Source: CAD feature listing. Evaluate the final solid. Frame: model axes, mm. Face numbers are marked on the shaded views. A direction names the side the tool comes from. Coordinates: 2 decimals unless noted, no trailing zeros. Write each loop counter-clockwise with the first axis right and the second up, starting at its lowest first coordinate (ties: lowest second). Pieces come first, ordered by that corner, then holes. Notation, with made-up numbers: (49.25, 35.25) - (95.25, 35.25) arc R18 cw to (95.25, 58.25) - close; hole circle Ø1 at (25.5, 40.25). An arc over 180 degrees is marked (long way). One line per item, written item: value.
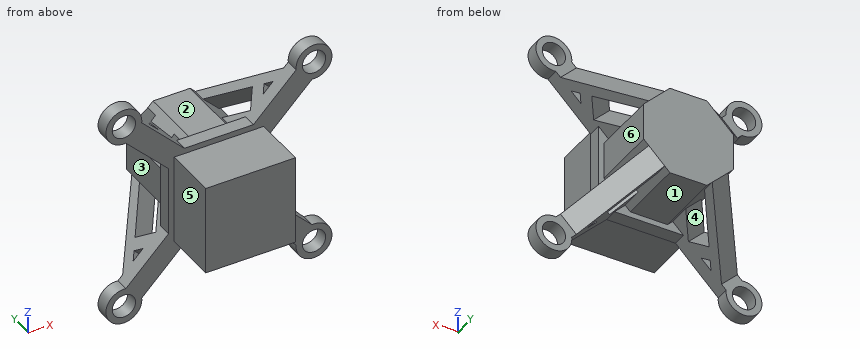
from build123d import *

# Parameters (mm, degrees)
SKETCH1_W               = 20
SKETCH1_H               = 20
BOSS_EXTRUDE1_DEPTH     = 12
BOSS_EXTRUDE2_DEPTH     = 3
BOSS_EXTRUDE3_DEPTH     = 15
BOSS_EXTRUDE4_DEPTH     = 15
BODY_MOVE_COPY1_ANGLE   = 45
CUT_EXTRUDE2_DEPTH      = 15
CUT_EXTRUDE2_DEPTH_BACK = 15
CUT_EXTRUDE3_DEPTH      = 15
CUT_EXTRUDE3_DEPTH_BACK = 15
CUT_EXTRUDE4_DEPTH      = 15
CUT_EXTRUDE4_DEPTH_BACK = 15
CUT_EXTRUDE5_DEPTH      = 15
CUT_EXTRUDE5_DEPTH_BACK = 15
SKETCH10_R              = 2.6
CUT_EXTRUDE6_DEPTH      = 25
BODY_MOVE_COPY2_ANGLE   = 45


with BuildPart() as part:
    # Sketch1 → Boss-Extrude1 (new body)
    with BuildSketch(Plane(origin=(0, 0, 0), x_dir=(1, 0, 0), z_dir=(0, 1, 0))):
        Rectangle(SKETCH1_W, SKETCH1_H)
    extrude(amount=-BOSS_EXTRUDE1_DEPTH)

    # Sketch2 → Boss-Extrude2 (add)
    with BuildSketch(Plane(origin=(0, 0, 0), x_dir=(1, 0, 0), z_dir=(0, 1, 0))):
        with BuildLine():
            Line((7.714466094, -11.25), (17.237496266, -20.773030172))
            ThreePointArc((17.237496266, -20.773030172), (24.04163056, -24.04163056), (20.773030172, -17.237496266))
            Line((20.773030172, -17.237496266), (11.25, -7.714466094))
            Line((11.25, -7.714466094), (11.25, 7.714466094))
            Line((11.25, 7.714466094), (20.773030172, 17.237496266))
            ThreePointArc((20.773030172, 17.237496266), (24.04163056, 24.04163056), (17.237496266, 20.773030172))
            Line((17.237496266, 20.773030172), (7.714466094, 11.25))
            Line((7.714466094, 11.25), (-7.714466094, 11.25))
            Line((-7.714466094, 11.25), (-17.237496266, 20.773030172))
            ThreePointArc((-17.237496266, 20.773030172), (-24.04163056, 24.04163056), (-20.773030172, 17.237496266))
            Line((-20.773030172, 17.237496266), (-11.25, 7.714466094))
            Line((-11.25, 7.714466094), (-11.25, -7.714466094))
            Line((-11.25, -7.714466094), (-20.773030172, -17.237496266))
            ThreePointArc((-20.773030172, -17.237496266), (-24.04163056, -24.04163056), (-17.237496266, -20.773030172))
            Line((-17.237496266, -20.773030172), (-7.714466094, -11.25))
            Line((-7.714466094, -11.25), (7.714466094, -11.25))
        make_face()
    extrude(amount=BOSS_EXTRUDE2_DEPTH)

    # Sketch3 → Boss-Extrude3 (add)
    with BuildSketch(Plane(origin=(0, 3, 0), x_dir=(1, 0, 0), z_dir=(0, 1, 0))):
        Polygon((10, 4.142135624), (4.142135624, 10), (-4.142135624, 10), (-10, 4.142135624), (-10, -4.142135624), (-4.142135624, -10), (4.142135624, -10), (10, -4.142135624), align=None)
    extrude(amount=BOSS_EXTRUDE3_DEPTH)

    # Sketch4 → Boss-Extrude4 (add)
    with BuildSketch(Plane(origin=(0, 3, 0), x_dir=(1, 0, 0), z_dir=(0, 1, 0))):
        Polygon((-11.25, -7.714466094), (-19.735281374, -16.199747468), (-16.199747468, -19.735281374), (-7.714466094, -11.25), (-5.303300859, -8.838834765), (-8.838834765, -5.303300859), align=None)
        Polygon((-7.714466094, 11.25), (-16.199747468, 19.735281374), (-19.735281374, 16.199747468), (-11.25, 7.714466094), (-8.838834765, 5.303300859), (-5.303300859, 8.838834765), align=None)
        Polygon((11.25, 7.714466094), (19.735281374, 16.199747468), (16.199747468, 19.735281374), (7.714466094, 11.25), (5.303300859, 8.838834765), (8.838834765, 5.303300859), align=None)
        Polygon((7.714466094, -11.25), (16.199747468, -19.735281374), (19.735281374, -16.199747468), (11.25, -7.714466094), (8.838834765, -5.303300859), (5.303300859, -8.838834765), align=None)
    extrude(amount=BOSS_EXTRUDE4_DEPTH)


with BuildPart() as part_1:
    # Body-Move/Copy1: moved
    add(part.part.rotate(Axis((0, 0, 0), (0, 1, 0)), BODY_MOVE_COPY1_ANGLE))

    # Sketch5 → Cut-Extrude2 (cut, two sides: drawn at the far end of the back side and taken through both)
    with BuildSketch(Plane.XY.offset(-CUT_EXTRUDE2_DEPTH_BACK)):
        Polygon((-25.409902577, 18), (-10, 18), (-25.409902577, 3), align=None)
        Polygon((10, 18), (25.409902577, 3), (25.409902577, 18), align=None)
    extrude(amount=CUT_EXTRUDE2_DEPTH + CUT_EXTRUDE2_DEPTH_BACK, mode=Mode.SUBTRACT)

    # Sketch7 → Cut-Extrude3 (cut, two sides: drawn at the far end of the back side and taken through both)
    with BuildSketch(Plane(origin=(0, 0, 0), x_dir=(0, 0, -1), z_dir=(1, 0, 0)).offset(-CUT_EXTRUDE3_DEPTH_BACK)):
        Polygon((-25.409902577, 18), (-10, 18), (-25.409902577, 3), align=None)
        Polygon((10, 18), (25.409902577, 3), (25.409902577, 18), align=None)
    extrude(amount=CUT_EXTRUDE3_DEPTH + CUT_EXTRUDE3_DEPTH_BACK, mode=Mode.SUBTRACT)

    # Sketch8 → Cut-Extrude4 (cut, two sides: drawn at the far end of the back side and taken through both)
    with BuildSketch(Plane(origin=(2.5, 0, 0), x_dir=(0, 0, -1), z_dir=(1, 0, 0)).offset(-CUT_EXTRUDE4_DEPTH_BACK)):
        Polygon((-10, 7.94465349), (-10, 15.084865647), (-18.514759568, 6.570106079), (-14.94465349, 3), align=None)
        Polygon((-18.955808103, 3), (-22.084865647, 3), (-20.674172955, 4.410692692), (-20.520336875, 4.564528772), align=None)
        Polygon((14.94465349, 3), (10, 7.94465349), (10, 15.084865647), (18.514759568, 6.570106079), align=None)
        Polygon((20.674172955, 4.410692692), (20.520336875, 4.564528772), (18.955808103, 3), (22.084865647, 3), align=None)
    extrude(amount=CUT_EXTRUDE4_DEPTH + CUT_EXTRUDE4_DEPTH_BACK, mode=Mode.SUBTRACT)

    # Sketch9 → Cut-Extrude5 (cut, two sides: drawn at the far end of the back side and taken through both)
    with BuildSketch(Plane.XY.offset(-CUT_EXTRUDE5_DEPTH_BACK)):
        Polygon((-10, 7.94465349), (-10, 15.084865647), (-18.514759568, 6.570106079), (-14.94465349, 3), align=None)
        Polygon((-18.955808103, 3), (-22.084865647, 3), (-20.674172955, 4.410692692), (-20.520336875, 4.564528772), align=None)
        Polygon((14.94465349, 3), (10, 7.94465349), (10, 15.084865647), (18.514759568, 6.570106079), align=None)
        Polygon((20.674172955, 4.410692692), (20.520336875, 4.564528772), (18.955808103, 3), (22.084865647, 3), align=None)
    extrude(amount=CUT_EXTRUDE5_DEPTH + CUT_EXTRUDE5_DEPTH_BACK, mode=Mode.SUBTRACT)

    # Sketch10 → Cut-Extrude6 (cut)
    with BuildSketch(Plane(origin=(0, 0, 0), x_dir=(1, 0, 0), z_dir=(0, 1, 0))):
        with Locations(Location((0, -30, 0), (0, 0, 270))):
            Circle(SKETCH10_R)
        with Locations(Location((-30, 0, 0), (0, 0, 270))):
            Circle(SKETCH10_R)
        with Locations(Location((0, 30, 0), (0, 0, 270))):
            Circle(SKETCH10_R)
        with Locations(Location((30, 0, 0), (0, 0, 270))):
            Circle(SKETCH10_R)
    extrude(amount=CUT_EXTRUDE6_DEPTH, mode=Mode.SUBTRACT)


with BuildPart() as part_2:
    # Body-Move/Copy2: moved
    add(part_1.part.rotate(Axis((0, 0, 0), (0, 1, 0)), BODY_MOVE_COPY2_ANGLE))


solid = part_2.part
1) Section query A-A on x = 2. Output: boundary loops of the cut face in (y, z), then the cut area to 4 significant figures.
Values found:
outline: (-12, -10) - (0, -10) - (0, -11.25) - (3, -11.25) - (3, -10) - (18, -10) - (18, 10) - (3, 10) - (3, 11.25) - (0, 11.25) - (0, 10) - (-12, 10) - close
area: 607.5 mm2
2) Reachability of the marked faces 4, 5 and 6 from +Z, -Z, +X, -X, +Y, -Y: full face, straight path, thin tool, end or side. Return the list, or none.
Values found:
face 4: none
face 5: +Z, -Z, -X, -Y
face 6: +X, +Y
3) Draft query along Z for the marked faces 1, 2 and 3. Return one class per face: released by +Z, released by -Z, zero draft, split by the parting line, or undercut.
Values found:
face 1: released by -Z
face 2: released by +Z
face 3: undercut
4) Section query D-D on y = 1.25. Output: boundary loops of the cut face in (x, z).
Values found:
outline: (-20.77, -17.24) arc R4 ccw (long way) to (-17.24, -20.77) - (-7.71, -11.25) - (7.71, -11.25) - (17.24, -20.77) arc R4 ccw (long way) to (20.77, -17.24) - (11.25, -7.71) - (11.25, 7.71) - (20.77, 17.24) arc R4 ccw (long way) to (17.24, 20.77) - (7.71, 11.25) - (-7.71, 11.25) - (-17.24, 20.77) arc R4 ccw (long way) to (-20.77, 17.24) - (-11.25, 7.71) - (-11.25, -7.71) - close; hole circle Ø5.2 at (-21.21, -21.21); hole circle Ø5.2 at (-21.21, 21.21); hole circle Ø5.2 at (21.21, -21.21); hole circle Ø5.2 at (21.21, 21.21)
5) Contact query for flat-ended pins moving along their axis: P1, Ø3, axis at x = 16, z = 13.5, coming from the +Y side; P2, Ø8.5, axis at x = 21.21, z = -21.21, coming from the +Y side; P3, Ø7, axis at x = 18.5, z = 21, coming from the +Y side; P4, Ø3, axis at x = 13, z = 1.5, coming from the -Y side. Output: stop coordinate, or through.
Values found:
P1: y = 8.89
P2: y = 3
P3: y = 3.95
P4: through
6) Section query C-C on z = 1.5. Output: boundary loops of the cut face in (x, y).
Values found:
outline: (-11.25, 0) - (-10, 0) - (-10, -12) - (10, -12) - (10, 0) - (11.25, 0) - (11.25, 3) - (10, 3) - (10, 18) - (-10, 18) - (-10, 3) - (-11.25, 3) - close
7) Section query B-B on y = 9. Output: boundary loops of the cut face in (x, z).
Values found:
outline: (-15.38, -11.84) - (-11.84, -15.38) - (-9.61, -13.14) - (-13.14, -9.61) - close; (-15.38, 11.84) - (-13.14, 9.61) - (-9.61, 13.14) - (-11.84, 15.38) - close; (-10, -4.14) - (-4.14, -10) - (4.14, -10) - (10, -4.14) - (10, 4.14) - (4.14, 10) - (-4.14, 10) - (-10, 4.14) - close; (9.61, -13.14) - (11.84, -15.38) - (15.38, -11.84) - (13.14, -9.61) - close; (9.61, 13.14) - (13.14, 9.61) - (15.38, 11.84) - (11.84, 15.38) - close
8) Material intervals for line 1 (Z direction, x = -21, y = 1.5); line 2 (X direction, y = 14.25, z = -7.5); line 3 (Z direction, x = 1, y = 9.5), sorted ascending.
Values found:
line 1: -25.21 to -23.8, -18.62 to -17.22, 17.22 to 18.62, 23.8 to 25.21
line 2: -11.04 to -7.82, -6.64 to 6.64, 7.82 to 11.04
line 3: -10 to 10
